Work out the finished part from the listing and answer in its coordinate system (mm). A direction names the side the tool comes from. Coordinates: 2 decimals unless noted, no trailing zeros. Write each loop counter-clockwise with the first axis right and the second up, starting at its lowest first coordinate (ties: lowest second). Pieces come first, ordered by that corner, then holes. Notation, with made-up numbers: (33.25, 82.25) - (39.25, 82.25) arc R8 cw to (39.25, 94.25) - close; hole circle Ø8 at (-39, 82.25). An arc over 180 degrees is marked (long way). One line per item, written item: value.
Autodesk Inventor part; units mm, degrees
ref_plane "Arbeitsebene1" through (0, -0.5, 0) normal (0, 1, 0) x (1, 0, 0)
ref_plane "YZ Plane" through (0, 0, 0) normal (1, 0, 0) x (0, 1, 0)
ref_plane "XZ Plane" through (0, 0, 0) normal (0, 1, 0) x (-1, 0, 0)
sketch "Skizze1" plane through (0, 0, 0) normal (0, 1, 0) x (-1, 0, 0)
  circle A0 centre (0, 0) radius 3.5
  line L0 (5.875, -5.875) -> (-5.875, -5.875)
  line L1 (-5.875, -5.875) -> (-5.875, 5.875)
  line L2 (-5.875, 5.875) -> (5.875, 5.875)
  line L3 (5.875, 5.875) -> (5.875, -5.875)
  line L4 (8.225, 0) -> (-8.225, 0)
  line L5 (0.75, 5.875) -> (-0.75, 5.875)
  line L6 (0, -8.225) -> (0, 8.225)
  point P0 (0.75, -5.875)
  point P1 (-5.875, -0.75)
  point P2 (5.875, -0.75)
  dimension "d1" = 7
  dimension "d2" = 11.75
  dimension "d3" = 11.75
extrude "Extrusion1" add sketch "Skizze1" along normal mid plane 3
sketch "Skizze2" plane through (0, 1.5, 0) normal (0, 1, 0) x (1, 0, 0)
  circle A0 centre (0, 0) radius 3
  dimension "d14" = 6
ref_plane "Arbeitsebene1" through (0, -0.5, 0) normal (0, 1, 0) x (1, 0, 0)
sketch "Skizze4" plane through (0, -1.5, 0) normal (0, -1, 0) x (1, 0, 0)
  circle A0 centre (0, 0) radius 3
  circle A1 centre (0, 0) radius 1.4
  circle A2 centre (0, 0) radius 4.1
  dimension "d20" = 6
  dimension "d21" = 8.2
extrude "Extrusion4" add sketch "Skizze4" along normal blind 3.5 contours A2
sketch "Skizze5" plane through (0, 1.5, 0) normal (0, 1, 0) x (1, 0, 0)
  line L0 (-5.875, 5.875) -> (5.875, 5.875)
  line L1 (-5.875, 5.875) -> (-3.775, 5.875)
  line L2 (-3.775, 5.875) -> (-3.775, 3.775)
  line L3 (-3.775, 3.775) -> (-5.875, 3.775)
  line L4 (-5.875, 3.775) -> (-5.875, 5.875)
  line L5 (-5.875, 5.875) -> (5.875, 5.875)
  line L6 (5.875, 5.875) -> (3.775, 5.875)
  line L7 (3.775, 5.875) -> (3.775, 3.775)
  line L8 (3.775, 3.775) -> (5.875, 3.775)
  line L9 (5.875, 3.775) -> (5.875, 5.875)
  line L10 (-5.875, -5.875) -> (-5.875, 5.875)
  line L11 (-5.875, -5.875) -> (-3.775, -5.875)
  line L12 (-3.775, -5.875) -> (-3.775, -3.775)
  line L13 (-3.775, -3.775) -> (-5.875, -3.775)
  line L14 (-5.875, -3.775) -> (-5.875, -5.875)
  line L15 (5.875, -5.875) -> (-5.875, -5.875)
  line L16 (5.875, -5.875) -> (3.775, -5.875)
  line L17 (3.775, -5.875) -> (3.775, -3.775)
  line L18 (3.775, -3.775) -> (5.875, -3.775)
  line L19 (5.875, -3.775) -> (5.875, -5.875)
  point P0 (0, 0)
  point P1 (-0.75, 5.75)
  point P2 (0.75, 5.75)
  point P3 (-5.75, -0.75)
  point P4 (0.75, -5.75)
  dimension "d24" = 2.1
  dimension "d25" = 2.1
  dimension "d26" = 2.1
  dimension "d27" = 2.1
  dimension "d28" = 2.1
  dimension "d29" = 2.1
  dimension "d30" = 2.1
  dimension "d31" = 2.1
extrude "Extrusion5" cut sketch "Skizze5" against normal blind 6
extrude "Extrusion6" cut sketch "Skizze2" against normal blind 1
sketch "Skizze6" plane through (0, 0.5, 0) normal (0, 1, 0) x (1, 0, 0)
  circle A0 centre (0, 0) radius 1.55
  dimension "d38" = 3.1
extrude "Extrusion7" cut sketch "Skizze6" against normal up to surface (2 mm away)
properties part number "_3D-Druck"
Item 1: Section A-A, the plane x = 0 is taken. Determine the outline of the cut face in (y, z) (3 decimals), then the cut area to 4 significant figures.
Evaluation:
outline: (-5, -4.1) - (-1.5, -4.1) - (-1.5, -5.875) - (1.5, -5.875) - (1.5, -3) - (0.5, -3) - (0.5, -1.55) - (-1.5, -1.55) - (-1.5, -3) - (-5, -3) - close; (-5, 3) - (-1.5, 3) - (-1.5, 1.55) - (0.5, 1.55) - (0.5, 3) - (1.5, 3) - (1.5, 5.875) - (-1.5, 5.875) - (-1.5, 4.1) - (-5, 4.1) - close
area: 30.75 mm2
Item 2: Given pin 1 (0.6 mm diameter, centred on y = -0.5, z = 4.5, fed in from -X) (3 decimals); pin 2 (0.6 mm diameter, centred on y = 0, z = 4.5, fed in from +X) (3 decimals); pin 3 (4 mm diameter, centred on x = 2.5, z = 0, fed in from +Y); pin 4 (1 mm diameter, centred on x = -4.5, y = 0, fed in from -Z) (3 decimals), each flat-ended and moving along its own axis, determine where each tip first touches the part or whether it passes through.
Evaluation:
pin 1: stops at x = -3.775
pin 2: stops at x = 3.775
pin 3: stops at y = 1.5
pin 4: stops at z = -3.775
Item 3: Section B-B, the plane z = 0 is taken. Determine the outline of the cut face in (x, y) (3 decimals), then the cut area to 4 significant figures.
Evaluation:
outline: (-5.875, -1.5) - (-4.1, -1.5) - (-4.1, -5) - (-3, -5) - (-3, -1.5) - (-1.55, -1.5) - (-1.55, 0.5) - (-3, 0.5) - (-3, 1.5) - (-5.875, 1.5) - close; (1.55, -1.5) - (3, -1.5) - (3, -5) - (4.1, -5) - (4.1, -1.5) - (5.875, -1.5) - (5.875, 1.5) - (3, 1.5) - (3, 0.5) - (1.55, 0.5) - close
area: 30.75 mm2
Item 4: Determine the mould class of faces 4 (the face through (5, 0, -3.775)), 5 (the face through (-1.3, -1.5, -1.3)), 6 (the face through (3.775, 0, 5)) for opening direction Z: +Z half, -Z half, draft (parallel to the pull), parting line (faces both ways), or undercut.
Evaluation:
face 4: -Z half
face 5: undercut
face 6: draft
Item 5: Consider probe 1 along X at (y, z) = (-0.25, 0) (3 decimals); probe 2 along Z at (x, y) = (0, -2.7). Determine where each line is inside the solid, lowest interval first.
Evaluation:
probe 1: x = -5.875 to -1.55, 1.55 to 5.875
probe 2: z = -4.1 to -3, 3 to 4.1
Item 6: Section D-D, the plane z = 2 is taken. Determine the outline of the cut face in (x, y) (3 decimals), then the cut area to 3 significant figures.
Evaluation:
outline: (-5.875, -1.5) - (-3.579, -1.5) - (-3.579, -5) - (-2.236, -5) - (-2.236, -1.5) - (2.236, -1.5) - (2.236, -5) - (3.579, -5) - (3.579, -1.5) - (5.875, -1.5) - (5.875, 1.5) - (2.236, 1.5) - (2.236, 0.5) - (-2.236, 0.5) - (-2.236, 1.5) - (-5.875, 1.5) - close
area: 40.2 mm2
Item 7: Which of the six approach directions +Z, -Z, +X, -X, +Y, -Y give full straight-line access (tool end or side, diameter ignored) to faces 1 (the face through (-3.775, 0, -5)), 2 (the face through (3.775, 0, -5)), 3 (the face through (5, 0, 3.775))?
Evaluation:
face 1: -Z, -X, +Y, -Y
face 2: -Z, +X, +Y, -Y
face 3: +Z, +X, +Y, -Y
Item 8: Section C-C, the plane y = 1 is taken. Determine the outline of the cut face in (x, z) (3 decimals), then the cut area to 3 significant figures.
Evaluation:
outline: (-5.875, -3.775) - (-3.775, -3.775) - (-3.775, -5.875) - (3.775, -5.875) - (3.775, -3.775) - (5.875, -3.775) - (5.875, 3.775) - (3.775, 3.775) - (3.775, 5.875) - (-3.775, 5.875) - (-3.775, 3.775) - (-5.875, 3.775) - close; hole circle Ø6 at (0, 0)
area: 92.1 mm2
